```python
from build123d import *

# Parameters (mm, degrees)
SKETCH1_R           = 37.5
SKETCH1_R_2         = 29.5
BOSS_EXTRUDE1_DEPTH = 5
SKETCH2_R           = 1.5
CUT_EXTRUDE1_DEPTH  = 11


with BuildPart() as part:
    # Sketch1 → Boss-Extrude1 (new body)
    with BuildSketch(Plane.XY):
        Circle(SKETCH1_R)
        Circle(SKETCH1_R_2, mode=Mode.SUBTRACT)
    extrude(amount=BOSS_EXTRUDE1_DEPTH)

    # Sketch2 → Cut-Extrude1 (cut)
    with BuildSketch(Plane(origin=(0, 0, 0), x_dir=(-1, 0, 0), z_dir=(0, 0, -1))):
        with Locations((-17.005, 29.453523983)):
            Circle(SKETCH2_R)
        with Locations((17.005, 29.453523983)):
            Circle(SKETCH2_R)
        with Locations((34.01, 0)):
            Circle(SKETCH2_R)
        with Locations((17.005, -29.453523983)):
            Circle(SKETCH2_R)
        with Locations((-17.005, -29.453523983)):
            Circle(SKETCH2_R)
        with Locations((-34.01, 0)):
            Circle(SKETCH2_R)
    extrude(amount=-CUT_EXTRUDE1_DEPTH, mode=Mode.SUBTRACT)


solid = part.part
```
Work out the finished part from the listing and answer in its coordinate system (mm). Round coordinates to 2 decimals unless told otherwise and drop trailing zeros. Write each loop counter-clockwise with the first axis right and the second up, starting at its lowest first coordinate (ties: lowest second). Pieces come first, ordered by that corner, then holes.
1) A cutting plane is placed at B-B on y = 0. Determine the outline of the cut face in (x, z), and give its area (3 significant figures).
2) Determine the mould class of faces 1 (the face through (-20, 22, 5)), 2 (the face through (-4.88, 37.18, 2.46)), 3 (the face through (16.2, 30.72, 2.46)) for opening direction Y: pulls with the +Y half, pulls with the -Y half, needs draft (parallel to the pull), parting line crosses it, or undercut.
3) A cutting plane is placed at C-C on y = -21. Determine the outline of the cut face in (x, z), and give its area (3 significant figures).
4) A cutting plane is placed at A-A on x = 0. Determine the outline of the cut face in (y, z), and give its area (3 significant figures).
5) Flat-ended cylindrical pins translate along their axes: P1, Ø3, axis at x = -28.5, y = -10, coming from the -Z side; P2, Ø1, axis at x = 19.5, z = 1.5, coming from the +Y side; P3, Ø3, axis at x = 18, z = 1, coming from the +Y side; P4, Ø3, axis at x = 15, z = 3, coming from the +Y side. Find the tip coordinate at first contact, or state that the pin passes through.
6) Consider probe 1 along Y at (x, z) = (0, 1); probe 2 along X at (y, z) = (22, 4.5); probe 3 along X at (y, z) = (25, 4.75). Determine where each line is inside the solid, lowest interval first.
Entries:
1. outline: (-37.5, 0) - (-35.51, 0) - (-35.51, 5) - (-37.5, 5) - close; (-32.51, 0) - (-29.5, 0) - (-29.5, 5) - (-32.51, 5) - close; (29.5, 0) - (32.51, 0) - (32.51, 5) - (29.5, 5) - close; (35.51, 0) - (37.5, 0) - (37.5, 5) - (35.51, 5) - close
1. area: 50.0 mm2
2. face 1: needs draft
2. face 2: parting line crosses it
2. face 3: undercut
3. outline: (-31.07, 0) - (-20.72, 0) - (-20.72, 5) - (-31.07, 5) - close; (20.72, 0) - (31.07, 0) - (31.07, 5) - (20.72, 5) - close
3. area: 104 mm2
4. outline: (-37.5, 0) - (-29.5, 0) - (-29.5, 5) - (-37.5, 5) - close; (29.5, 0) - (37.5, 0) - (37.5, 5) - (29.5, 5) - close
4. area: 80.0 mm2
5. P1: stops at z = 0
5. P2: stops at y = 32.33
5. P3: stops at y = 33.67
5. P4: stops at y = 34.99
6. probe 1: y = -37.5 to -29.5, 29.5 to 37.5
6. probe 2: x = -30.37 to -19.65, 19.65 to 30.37
6. probe 3: x = -27.95 to -15.66, 15.66 to 27.95
